from build123d import *

# Parameters (mm, degrees)
BOSS_EXTRUDE1_DEPTH      = 350
BOSS_EXTRUDE2_DEPTH      = 50
SKETCH3_W                = 50
SKETCH3_H                = 24.508106186
BOSS_EXTRUDE3_DEPTH      = 90
SKETCH4_W                = 49.133865319
SKETCH4_H                = 39.302733228
SKETCH4_W_2              = 45.648473343
BOSS_EXTRUDE4_DEPTH      = 30
BOSS_EXTRUDE5_DEPTH      = 50
BOSS_EXTRUDE5_DEPTH_BACK = 40
SKETCH5_W                = 13.251857059
SKETCH5_H                = 52.991624954
SKETCH5_W_2              = 15.951284084
SKETCH5_H_2              = 35.82978704
BOSS_EXTRUDE6_DEPTH      = 50
BOSS_EXTRUDE6_DEPTH_BACK = 50
SKETCH6_W                = 13.251857059
SKETCH6_H                = 52.991624954


with BuildPart() as part:
    # Sketch1 → Boss-Extrude1 (new body)
    with BuildSketch(Plane(origin=(0, 0, 0), x_dir=(0, 0, -1), z_dir=(1, 0, 0))):
        Polygon((0, 0), (1229.23703731, -216.747655364), (1211.872219543, -315.228430665), (-17.364817767, -98.480775301), align=None)
    extrude(amount=BOSS_EXTRUDE1_DEPTH)

    # Sketch2 → Boss-Extrude2 (add)
    with BuildSketch(Plane(origin=(350, 0, 0), x_dir=(0, 0, -1), z_dir=(1, 0, 0))):
        Polygon((-17.364817767, -98.480775301), (46.338371166, 262.797961946), (1275.575408476, 46.050306583), (1211.872219543, -315.228430665), align=None)
    extrude(amount=BOSS_EXTRUDE2_DEPTH)

    # Sketch3 → Boss-Extrude3 (add)
    with BuildSketch(Plane(origin=(0, -216.747655364, -1229.23703731), x_dir=(-1, 0, 0), z_dir=(0, -0.17364817766693216, -0.9848077530122078))):
        with Locations((-375, 254.597991017)):
            Rectangle(SKETCH3_W, SKETCH3_H)
    extrude(amount=BOSS_EXTRUDE3_DEPTH)

    # Sketch4 → Boss-Extrude4 (add)
    with BuildSketch(Plane(origin=(0, 0, 0), x_dir=(1, 0, 0), z_dir=(0, 0.17364817766693608, 0.9848077530122071))):
        with Locations((96.899550705, -19.651366614)):
            Rectangle(SKETCH4_W, SKETCH4_H)
        with Locations((362.077115008, -19.651366614)):
            Rectangle(SKETCH4_W_2, SKETCH4_H)
    extrude(amount=BOSS_EXTRUDE4_DEPTH)

    # Sketch5 → Boss-Extrude5 (add, two sides: drawn at the far end of the back side and taken through both)
    with BuildSketch(Plane(origin=(384.901351679, 0, 0), x_dir=(0, 0, -1), z_dir=(1, 0, 0)).offset(-BOSS_EXTRUDE5_DEPTH_BACK)):
        with Locations((-28.222892828, -9.605101255)):
            Rectangle(SKETCH5_W, SKETCH5_H)
        with Locations((1357.200809648, 15.148973405)):
            Rectangle(SKETCH5_W_2, SKETCH5_H_2)
    extrude(amount=BOSS_EXTRUDE5_DEPTH + BOSS_EXTRUDE5_DEPTH_BACK)

    # Sketch6 → Boss-Extrude6 (add, two sides: drawn at the far end of the back side and taken through both)
    with BuildSketch(Plane(origin=(121.466483364, 0, 0), x_dir=(0, 0, -1), z_dir=(1, 0, 0)).offset(-BOSS_EXTRUDE6_DEPTH_BACK)):
        with Locations((-28.222892828, -9.605101255)):
            Rectangle(SKETCH6_W, SKETCH6_H)
    extrude(amount=BOSS_EXTRUDE6_DEPTH + BOSS_EXTRUDE6_DEPTH_BACK)


solid = part.part
Build history of the part. All positions in model axes, mm. A direction names the side the tool comes from. Give positions to 0.01 mm unless a question says otherwise; leave off trailing zeros. Write each loop counter-clockwise with the first axis right and the second up, starting at its lowest first coordinate (ties: lowest second). Pieces come first, ordered by that corner, then holes. Notation, with made-up numbers: (12, 44) - (37, 44) arc R20 ccw to (37, 82) - close; hole circle Ø4 at (89.5, -8). An arc over 180 degrees is marked (long way). Use one line per item in the form item = value. Start each with the question number.
1. Band-saw the part on B-B on z = -824.5. Write the cut outline in (x, y).
2. 3-axis set-ups, long thin cutter, end or side, ignore diameter. For faces 5 (the face through (399, -4, 21.597)), 6 (the face through (339.253, -17, 18)), 7 (the face through (143, -4, 21.597)): which of +Z, -Z, +X, -X, +Y, -Y reach the whole face in a straight line?
3. Two-plate mould, pull along X, no slides. Class faces 1 (the face through (356.899, -25.521, 34.963)), 2 (the face through (389, -10, 34.849)), 3 (the face through (400, -34, -658)), 4 (the face through (0, -145, -609)): released by +X, released by -X, zero draft, split by the parting line, or undercut.
4. Band-saw the part on C-C on y = -128. Write the cut outline in (x, z), plus the area to 3 significant figures.
5. Probe line 1 (X direction, y = 30.5, z = -157.5); line 2 (X direction, y = -175.5, z = -828); line 3 (Y direction, x = 241.5, z = -720.5). List the from-to ranges inside material, lowest first. Write a range as [from, to].
6. Band-saw the part on A-A on x = 97. Write the cut outline in (y, z), plus the area to 3 significant figures.
7. Drop flat-ended pins along their axis: pin 1 Ø10.5 at (y, z) = (-4.5, 26.5) entering from -X; pin 2 Ø17.5 at (y, z) = (-17.5, 6) entering from +X; pin 3 Ø3 at (x, z) = (268.5, -1153) entering from +Y. Give the stop position or say it passes through.
8. Band-saw the part on D-D on x = 199.5. Write the cut outline in (y, z).
Conclusion:
q1.outline = (0, -246.92) - (400, -246.92) - (400, 125.59) - (350, 125.59) - (350, -145.38) - (0, -145.38) - close
q2.face_5 = +X, +Y
q2.face_6 = +Z, +Y
q2.face_7 = +Y
q3.face_1 = undercut
q3.face_2 = zero draft
q3.face_3 = released by +X
q3.face_4 = released by -X
q4.outline = (0, -725.92) - (350, -725.92) - (350, -1244.89) - (400, -1244.89) - (400, -150.05) - (0, -150.05) - close
q4.area = 256,000 mm²
q5.line_1 = [350, 400]
q5.line_2 = [0, 400]
q5.line_3 = [-228.59, -127.04]
q6.outline = (-315.23, -1211.87) - (-216.75, -1229.24) - (3.81, 21.6) - (16.89, 21.6) - (16.89, 34.85) - (-24.87, 34.85) - (-33.5, 36.37) - (-33.76, 34.85) - (-36.1, 34.85) - (-36.1, 21.6) - (-38.71, 6.82) - (-98.48, 17.36) - close
q6.area = 126,000 mm²
q7.pin_1 = 71.47
q7.pin_2 = 400
q7.pin_3 = -203.04
q8.outline = (-315.23, -1211.87) - (-216.75, -1229.24) - (0, 0) - (-98.48, 17.36) - close
